Build history of the part. All positions in model axes, mm. Face numbers are marked on the shaded views. A direction names the side the tool comes from. Round coordinates to 2 decimals unless told otherwise and drop trailing zeros. Loops run counter-clockwise (first coordinate to the right, second up) from the corner with the lowest first, then second, coordinate; pieces in that order, holes last. Notation, with made-up numbers: (-2, 76.5) -> (44, 76.5) arc R17 cw to (44, 89.5) -> close; hole circle Ø2 at (34, 25.25). An arc over 180 degrees is marked (long way). Put each result on its own line as item: value. Start each with the question number.
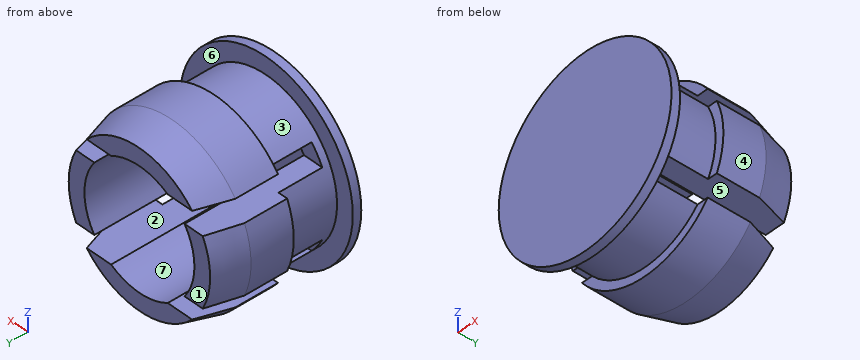
```python
from build123d import *

# Parameters (mm, degrees)
CROQUIS2_W            = 26
CROQUIS2_H            = 2
CORTAR_EXTRUIR1_DEPTH = 14


with BuildPart() as part:
    # Croquis1 → Revolución1 (revolve)
    with BuildSketch(Plane.XY):
        Polygon((-89.778094977, -14.637996222), (-78.782252338, -14.637996222), (-78.782252338, -13.637996222), (-85.782252338, -13.637996222), (-85.782252338, 1.235955759), (-87.782252338, 1.235955759), (-88.782252338, -2.637996222), (-88.782252338, -7.637996222), (-87.782252338, -7.637996222), (-87.782252338, -13.637996222), (-89.778094977, -13.637996222), align=None)
    revolve(axis=Axis((-78.782252338, -14.637996222, 0), (0, 1, 0)))

    # Croquis2 → Cortar-Extruir1 (cut)
    with BuildSketch(Plane(origin=(0, 1.235955759, 0), x_dir=(1, 0, 0), z_dir=(0, 1, 0))):
        with Locations((-78.782252338, -5)):
            Rectangle(CROQUIS2_W, CROQUIS2_H)
        with Locations((-78.782252338, 5)):
            Rectangle(CROQUIS2_W, CROQUIS2_H)
    extrude(amount=-CORTAR_EXTRUIR1_DEPTH, mode=Mode.SUBTRACT)


solid = part.part
```
Item 1: 3-axis set-ups, long thin cutter, end or side, ignore diameter. For the marked faces 4, 5, 6 and 7: which of +Z, -Z, +X, -X, +Y, -Y reach the whole face in a straight line?
Item 2: Pull direction Z, two halves, no side cores. Call the marked faces 1, 2 and 3: +Z half, -Z half, draft (parallel to the pull), parting line (faces both ways), or undercut.
Item 3: Cut at A-A on y = -6.5. Write the cut outline in (x, z), then the cut area to 3 significant figures.
Item 4: Cut at B-B on z = 0. Write the cut outline in (x, y), then the cut area to 3 significant figures.
Item 5: Drop flat-ended pins along their axis: pin 1 (6.5 mm diameter, centred on x = -79, z = 3, fed in from +Y); pin 2 (0.6 mm diameter, centred on x = -85.5, z = -5, fed in from +Y); pin 3 (2 mm diameter, centred on x = -84, y = -7.5, fed in from -Z). Give the stop position or say it passes through.
Item 6: Cut at D-D on x = -71.5. State how many separate pieces and enclosed holes the cut face has, then the cut area to 3 significant figures.
Item 7: Wall check: line 1 (Z direction, x = -72.5, y = -10); line 2 (X direction, y = -10, z = 0); line 3 (Y direction, x = -85, z = -0.5). Give the ranges that are in metal, low to high. Write a range as from..to.
Item 8: Cut at C-C on y = -11.5. Write the cut outline in (x, z).
Ans:
1. face 4: +X, +Y
1. face 5: +X, -X, +Y
1. face 6: none
1. face 7: +Y
2. face 1: draft
2. face 2: undercut
2. face 3: parting line
3. outline: (-87.95, -4) -> (-84.53, -4) arc R7 cw to (-84.53, 4) -> (-87.95, 4) arc R10 ccw to start; (-86.78, -6) arc R10 ccw to (-70.78, -6) -> (-75.18, -6) arc R7 cw to (-82.39, -6) -> close; (-86.78, 6) -> (-82.39, 6) arc R7 cw to (-75.18, 6) -> (-70.78, 6) arc R10 ccw to start; (-73.04, -4) -> (-69.62, -4) arc R10 ccw to (-69.62, 4) -> (-73.04, 4) arc R7 cw to start
3. area: 130 mm2
4. outline: (-89.78, -14.64) -> (-67.79, -14.64) -> (-67.79, -13.64) -> (-69.78, -13.64) -> (-69.78, -7.64) -> (-68.78, -7.64) -> (-68.78, -2.64) -> (-69.78, 1.24) -> (-71.78, 1.24) -> (-71.78, -13.64) -> (-85.78, -13.64) -> (-85.78, 1.24) -> (-87.78, 1.24) -> (-88.78, -2.64) -> (-88.78, -7.64) -> (-87.78, -7.64) -> (-87.78, -13.64) -> (-89.78, -13.64) -> close
4. area: 95.4 mm2
5. pin 1: stops at y = -13.64
5. pin 2: stops at y = -12.76
5. pin 3: stops at z = -9.07
6. separate pieces: 3
6. enclosed holes: 0
6. area: 148 mm2
7. line 1: z = -6.44..-6, -4..-3.09, 3.09..4, 6..6.44
7. line 2: x = -87.78..-85.78, -71.78..-69.78
7. line 3: y = -14.64..-13.64
8. outline: (-86.84, -4) -> (-84.53, -4) arc R7 cw to (-84.53, 4) -> (-86.84, 4) arc R9 ccw to start; (-85.49, -6) arc R9 ccw to (-72.07, -6) -> (-75.18, -6) arc R7 cw to (-82.39, -6) -> close; (-85.49, 6) -> (-82.39, 6) arc R7 cw to (-75.18, 6) -> (-72.07, 6) arc R9 ccw to start; (-73.04, -4) -> (-70.72, -4) arc R9 ccw to (-70.72, 4) -> (-73.04, 4) arc R7 cw to start
